The figure shows three views and two pictorial views of one solid part (mm, origin at its lowest corner). Answer the questions. A direction names the side the tool comes from. Coordinates: 2 decimals unless noted, no trailing zeros. Write each loop counter-clockwise with the first axis right and the second up, starting at its lowest first coordinate (ties: lowest second). Pieces come first, ordered by that corner, then holes.
Item 1: A tool of negligible diameter and unlimited length cuts with its end or side. For the marked faces 1 and 2, from which of +Z, -Z, +X, -X, +Y, -Y can it reach the whole face along a straight path? Write none if from no direction.
Item 2: Section B-B (y = 4.5) is taken. Give the vertices of the cut face in (x, z).
Item 3: Each of these flat-tipped pins is pushed along its axis until it touches: P1, Ø2.5, axis at x = 36.65, z = 5.65, coming from the +Y side; P2, Ø12, axis at x = 22.5, z = 29.5, coming from the +Y side; P3, Ø12, axis at x = 27.5, y = 27, coming from the -Z side. Where does it stop, or does it pass through?
Item 4: Determine the mould class of the marked faces 3, 4 and 5 for opening direction Z: released by +Z, released by -Z, zero draft, split by the parting line, or undercut.
Item 5: Straight lines are drawn through the part: probe 1 along Z at (x, y) = (5.65, 3.25); probe 2 along X at (y, z) = (2.75, 5.65); probe 3 along X at (y, z) = (12.5, 23.5). For each, find the intervals that lie inside material, in ascending order.
Item 6: Section C-C (x = 5.65) is taken. Give the vertices of the cut face in (y, z), then the cut area to 3 significant figures.
Item 7: Section A-A (x = 21.15) is taken. Give the vertices of the cut face in (y, z), then the cut area to 3 significant figures.
Item 8: Section D-D (z = 5.65) is taken. Give the vertices of the cut face in (x, y).
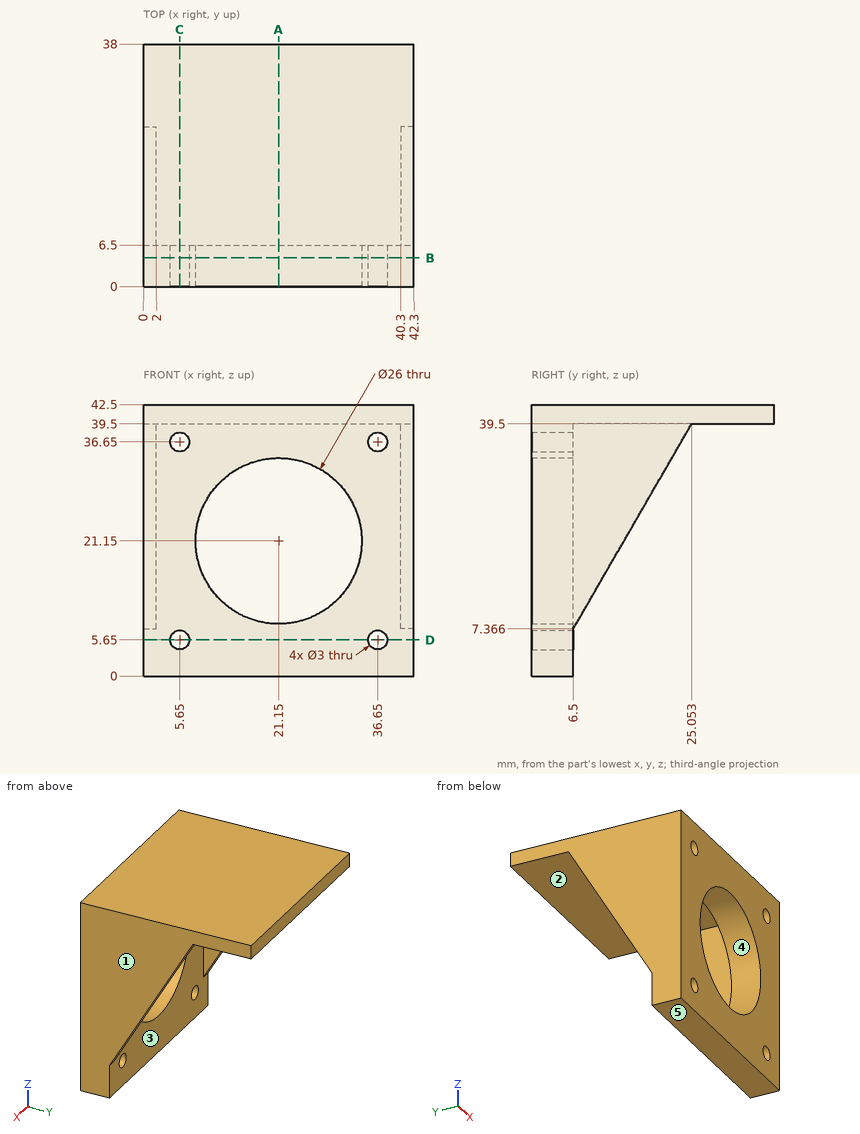
Established:
1. face 1: +Z, -Z, +X, +Y, -Y
1. face 2: -Z, +Y
2. outline: (0, 0) - (42.3, 0) - (42.3, 42.5) - (0, 42.5) - close; hole circle Ø3 at (5.65, 5.65); hole circle Ø3 at (5.65, 36.65); hole circle Ø26 at (21.15, 21.15); hole circle Ø3 at (36.65, 5.65); hole circle Ø3 at (36.65, 36.65)
3. P1: passes through
3. P2: stops at y = 6.5
3. P3: stops at z = 39.5
4. face 3: zero draft
4. face 4: undercut
4. face 5: released by -Z
5. probe 1: z = 0 to 4.15, 7.15 to 35.15, 38.15 to 42.5
5. probe 2: x = 0 to 4.15, 7.15 to 35.15, 38.15 to 42.3
5. probe 3: x = 0 to 2, 40.3 to 42.3
6. outline: (0, 0) - (6.5, 0) - (6.5, 4.15) - (0, 4.15) - close; (0, 7.15) - (6.5, 7.15) - (6.5, 35.15) - (0, 35.15) - close; (0, 38.15) - (6.5, 38.15) - (6.5, 39.5) - (38, 39.5) - (38, 42.5) - (0, 42.5) - close
6. area: 332 mm2
7. outline: (0, 0) - (6.5, 0) - (6.5, 8.15) - (0, 8.15) - close; (0, 34.15) - (6.5, 34.15) - (6.5, 39.5) - (38, 39.5) - (38, 42.5) - (0, 42.5) - close
7. area: 202 mm2
8. outline: (0, 0) - (4.15, 0) - (4.15, 6.5) - (0, 6.5) - close; (7.15, 0) - (35.15, 0) - (35.15, 6.5) - (7.15, 6.5) - close; (38.15, 0) - (42.3, 0) - (42.3, 6.5) - (38.15, 6.5) - close
